from build123d import *

# Parameters (mm, degrees)
SKETCH_1_W                     = 31
SKETCH_1_H                     = 40
SKETCH_1_R                     = 1.6
EXTRUDE_1_DEPTH                = 5
SKETCH_2_W                     = 31
SKETCH_2_H                     = 9.8
EXTRUDE_3_DEPTH                = 8
SKETCH_13_R                    = 1
CUT_EXTRUDE_7_DEPTH            = 5
EXTRUDE_START                  = 1
SKETCH_14_R                    = 3
SKETCH_14_R_2                  = 1
EXTRUDE_8_DEPTH                = 1
HOLE_WIZARD_M3_3_D             = 2.5
HOLE_WIZARD_M3_3_DEPTH         = 6.5
HOLE_WIZARD_M3_3_TIP           = 0.751075774
SKETCH_18_W                    = 31
SKETCH_18_H                    = 3
EXTRUDE_9_DEPTH                = 10
SKETCH_29_W                    = 31
SKETCH_29_H                    = 6.8
EXTRUDE_11_DEPTH               = 2
SKETCH_20_R                    = 1
CUT_EXTRUDE_9_DEPTH            = 9
HOLE_START                     = -9
HOLE_WIZARD_M3_1_OUTLINE_R     = 1.25
HOLE_WIZARD_M3_1_OUTLINE_R_2   = 1
HOLE_WIZARD_M3_1_DEPTH         = 9
HOLE_WIZARD_M3_1_3_D           = 3.2
HOLE_WIZARD_M3_1_3_CBORE_D     = 6
HOLE_WIZARD_M3_1_3_CBORE_DEPTH = 3.1
HOLE_START_2                   = -40
HOLE_WIZARD_M3_2_OUTLINE_R     = 1.25
HOLE_WIZARD_M3_2_OUTLINE_R_2   = 1
HOLE_WIZARD_M3_2_DEPTH         = 9
SKETCH_30_W                    = 31
SKETCH_30_H                    = 7
CUT_EXTRUDE_10_DEPTH           = 4
FILLET_3_R                     = 1


# Read off the part's stored shape, not the designer's step: M3 螺纹孔1, M3 螺纹孔2
with BuildPart() as part:
    # 草图1 → 凸台-拉伸1 (new body)
    with BuildSketch(Plane(origin=(0, 0, 0), x_dir=(1, 0, 0), z_dir=(0, 1, 0))):
        with Locations((15.5, 20)):
            Rectangle(SKETCH_1_W, SKETCH_1_H)
        with Locations(Location((20.5, 27.5, 0), (0, 0, 270))):
            Circle(SKETCH_1_R, mode=Mode.SUBTRACT)
        with Locations(Location((10.5, 27.5, 0), (0, 0, 270))):
            Circle(SKETCH_1_R, mode=Mode.SUBTRACT)
        with Locations(Location((10.5, 12.5, 0), (0, 0, 90))):
            Circle(SKETCH_1_R, mode=Mode.SUBTRACT)
        with Locations(Location((20.5, 12.5, 0), (0, 0, 90))):
            Circle(SKETCH_1_R, mode=Mode.SUBTRACT)
    extrude(amount=EXTRUDE_1_DEPTH)

    # 草图2 → 凸台-拉伸3 (add)
    with BuildSketch(Plane(origin=(0, 0, 0), x_dir=(1, 0, 0), z_dir=(0, 1, 0))):
        with Locations((15.5, 35.1)):
            Rectangle(SKETCH_2_W, SKETCH_2_H)
    extrude(amount=-EXTRUDE_3_DEPTH)

    # 草图13 → 切除-拉伸7 (cut)
    with BuildSketch(Plane.XZ.offset(8)):
        with Locations(Location((15.5, -35.1, 0), (0, 0, 270))):
            Circle(SKETCH_13_R)
    extrude(amount=-CUT_EXTRUDE_7_DEPTH, mode=Mode.SUBTRACT)

    # 草图14 → 凸台-拉伸8 (add)
    with BuildSketch(Plane.XZ.offset(8).offset(EXTRUDE_START)):
        with Locations(Location((15.5, -35.1, 0), (0, 0, 270))):
            Circle(SKETCH_14_R)
        with Locations(Location((15.5, -35.1, 0), (0, 0, 270))):
            Circle(SKETCH_14_R_2, mode=Mode.SUBTRACT)
    extrude(amount=-EXTRUDE_8_DEPTH)

    # M3 螺纹孔3
    with Locations(Plane(origin=(0, -9, 0), x_dir=(-1, 0, 0), z_dir=(0, -1, 0))):
        with Locations((-15.5, 35.1)):
            Hole(HOLE_WIZARD_M3_3_D / 2, depth=HOLE_WIZARD_M3_3_DEPTH)
            with Locations((0, 0, -(HOLE_WIZARD_M3_3_DEPTH + HOLE_WIZARD_M3_3_TIP / 2))):  # 118° drill point
                Cone(0, HOLE_WIZARD_M3_3_D / 2, HOLE_WIZARD_M3_3_TIP, mode=Mode.SUBTRACT)

    # 草图18 → 凸台-拉伸9 (add)
    with BuildSketch(Plane(origin=(0, 5, 0), x_dir=(1, 0, 0), z_dir=(0, 1, 0))):
        with Locations((15.5, 8.3)):
            Rectangle(SKETCH_18_W, SKETCH_18_H)
    extrude(amount=-EXTRUDE_9_DEPTH)

    # 草图29 → 凸台-拉伸11 (add)
    with BuildSketch(Plane.XZ):
        with Locations((15.5, -3.4)):
            Rectangle(SKETCH_29_W, SKETCH_29_H)
    extrude(amount=EXTRUDE_11_DEPTH)

    # 草图20 → 切除-拉伸9 (cut)
    with BuildSketch(Plane.XY):
        with Locations((7.5, 2)):
            Circle(SKETCH_20_R)
        with Locations(Location((23.5, 2, 0), (0, 0, 180))):
            Circle(SKETCH_20_R)
    cut_extrude_9 = extrude(amount=-CUT_EXTRUDE_9_DEPTH, mode=Mode.SUBTRACT)

    # Hole Wizard M3 _1 outline → Hole Wizard M3 _1 (cut)
    with BuildSketch(Plane.XY.offset(HOLE_START)):
        with Locations((23.5, 2)):
            Circle(HOLE_WIZARD_M3_1_OUTLINE_R)
        with Locations((23.5, 2)):
            Circle(HOLE_WIZARD_M3_1_OUTLINE_R_2, mode=Mode.SUBTRACT)
    extrude(amount=HOLE_WIZARD_M3_1_DEPTH, mode=Mode.SUBTRACT)

    # Hole Wizard M3 _1 2 outline → Hole Wizard M3 _1 2 (revolve, cut)
    with BuildSketch(Plane(origin=(7.5, 2, 0), x_dir=(1, 0, 0), z_dir=(0, -1, 0))):
        Polygon((0, -9), (0, -9.751075774), (1.25, -9), (1.25, 0), (1, 0), (1, -9), align=None)
    revolve(axis=Axis((7.5, 2, 0), (0, 0, 1)), mode=Mode.SUBTRACT)

    # 镜向1: 切除-拉伸9 across plane
    add(cut_extrude_9.mirror(Plane.XY.offset(-20)), mode=Mode.SUBTRACT)

    # Hole Wizard M3 _1 3 (through all)
    with Locations(Plane(origin=(0, 5, 0), x_dir=(1, 0, 0), z_dir=(0, 1, 0))):
        with Locations((10.5, 27.5), (10.5, 12.5), (20.5, 12.5), (20.5, 27.5)):
            CounterBoreHole(HOLE_WIZARD_M3_1_3_D / 2, HOLE_WIZARD_M3_1_3_CBORE_D / 2, HOLE_WIZARD_M3_1_3_CBORE_DEPTH)

    # M3 螺纹孔2 outline → M3 螺纹孔2 (cut)
    with BuildSketch(Plane.XY.offset(HOLE_START_2)):
        with Locations((7.5, 2)):
            Circle(HOLE_WIZARD_M3_2_OUTLINE_R)
        with Locations((7.5, 2)):
            Circle(HOLE_WIZARD_M3_2_OUTLINE_R_2, mode=Mode.SUBTRACT)
    extrude(amount=HOLE_WIZARD_M3_2_DEPTH, mode=Mode.SUBTRACT)

    # Hole Wizard M3 _2 2 outline → Hole Wizard M3 _2 2 (revolve, cut)
    with BuildSketch(Plane(origin=(23.5, 2, 0), x_dir=(1, 0, 0), z_dir=(0, -1, 0))):
        Polygon((1.25, -31), (0, -30.248924226), (0, -31), (1, -31), (1, -40), (1.25, -40), align=None)
    revolve(axis=Axis((23.5, 2, 0), (0, 0, 1)), mode=Mode.SUBTRACT)

    # 草图30 → 切除-拉伸10 (cut)
    with BuildSketch(Plane.XY):
        with Locations((15.5, 1.5)):
            Rectangle(SKETCH_30_W, SKETCH_30_H)
    cut_extrude_10 = extrude(amount=-CUT_EXTRUDE_10_DEPTH, mode=Mode.SUBTRACT)

    # 镜向3: 切除-拉伸10 across plane
    add(cut_extrude_10.mirror(Plane.XY.offset(-20)), mode=Mode.SUBTRACT)

    # 圆角3
    fillet_3_edges = [part.edges().sort_by_distance(p)[0] for p in [
        (31, 1.5, -4),
        (0, 1.5, -4),
        (31, -5, -40),
        (0, -5, -40),
        (0, 1.5, -36),
        (31, 1.5, -36),
        (31, -5, -8.3),
        (0, -5, -8.3),
    ]]
    fillet(fillet_3_edges, radius=FILLET_3_R)


solid = part.part
The listing builds one solid part. Answer for the finished solid, in the listing's coordinates (mm). A direction names the side the tool comes from. Give positions to 0.01 mm unless a question says otherwise; leave off trailing zeros. Write each loop counter-clockwise with the first axis right and the second up, starting at its lowest first coordinate (ties: lowest second). Pieces come first, ordered by that corner, then holes.
Item 1: Section C-C, the plane y = -6 is taken. Write down the section's boundary in (x, z).
Item 2: Find the intervals of material crossed by line 1 along X through (y, z) = (3.45, -12.5); line 2 along X through (y, z) = (1.05, -27.5); line 3 along Z through (x, y) = (10.5, 2.8), in increasing order.
Item 3: Determine the mould class of faces 5 (the cylindrical face through (6.25, 2.05, -6.46)), 6 (the cylindrical face through (30.699, -5.042, -39.715)), 7 (the cylindrical face through (21.58, 0.94, -28.68)) for opening direction Z: released by +Z, released by -Z, zero draft, split by the parting line, or undercut.
Item 4: Flat-ended cylindrical pins translate along their axes: P1, Ø1, axis at x = 7.5, y = -1, coming from the -Z side; P2, Ø10, axis at x = 16, z = -23.5, coming from the -Y side; P3, Ø0.8, axis at x = 17.5, z = -5.5, coming from the -Y side. Find the tip coordinate at first contact, or state that the pin passes through.
Item 5: Section B-B, the plane z = -12.5 is taken. Write down the section's boundary in (x, y), plus the area to 3 significant figures.
Item 6: Which of the six approach directions +Z, -Z, +X, -X, +Y, -Y give full straight-line access (tool end or side, diameter ignored) to faces 1 (the flat face through (15, -2, -9.8)), 2 (the cylindrical face through (30.699, -4.715, -8.321)), 3 (the flat face through (15, -2, -5)), 4 (the cylindrical face through (6.25, 2.05, -33.53))?
Item 7: Section A-A, the plane x = 20.5 is taken. Write down the section's boundary in (y, z), plus the area to 3 significant figures.
Item 8: Section D-D, the plane x = 27.5 is taken. Write down the section's boundary in (y, z), plus the area to 3 significant figures.
Completed:
1. outline: (0, -39) arc R1 ccw to (1, -40) - (30, -40) arc R1 ccw to (31, -39) - (31, -30.2) - (0, -30.2) - close; hole circle Ø2.5 at (15.5, -35.1)
2. line 1: x = 0 to 7.5, 13.5 to 17.5, 23.5 to 31
2. line 2: x = 0 to 8.9, 12.1 to 18.9, 22.1 to 31
2. line 3: z = -36 to -30.5, -24.5 to -15.5, -9.5 to -4
3. face 5: zero draft
3. face 6: released by -Z
3. face 7: undercut
4. P1: stops at z = -36
4. P2: stops at y = 0
4. P3: stops at y = -2
5. outline: (0, 0) - (8.9, 0) - (8.9, 1.9) - (7.5, 1.9) - (7.5, 5) - (0, 5) - close; (12.1, 0) - (18.9, 0) - (18.9, 1.9) - (17.5, 1.9) - (17.5, 5) - (13.5, 5) - (13.5, 1.9) - (12.1, 1.9) - close; (22.1, 0) - (31, 0) - (31, 5) - (23.5, 5) - (23.5, 1.9) - (22.1, 1.9) - close
5. area: 106 mm2
6. face 1: +X, -X, -Y
6. face 2: +Z, +X, -Y
6. face 3: +Z, +X, -X, -Y
6. face 4: -Z
7. outline: (-8, -40) - (-2, -40) - (-2, -36) - (5, -36) - (5, -30.5) - (1.9, -30.5) - (1.9, -29.1) - (0, -29.1) - (0, -30.2) - (-8, -30.2) - close; (-5, -9.8) - (0, -9.8) - (0, -10.9) - (1.9, -10.9) - (1.9, -9.5) - (5, -9.5) - (5, -4) - (-2, -4) - (-2, -6.8) - (-5, -6.8) - close; (0, -25.9) - (1.9, -25.9) - (1.9, -24.5) - (5, -24.5) - (5, -15.5) - (1.9, -15.5) - (1.9, -14.1) - (0, -14.1) - close
7. area: 202 mm2
8. outline: (-8, -40) - (-2, -40) - (-2, -36) - (5, -36) - (5, -4) - (-2, -4) - (-2, -6.8) - (-5, -6.8) - (-5, -9.8) - (0, -9.8) - (0, -30.2) - (-8, -30.2) - close
8. area: 251 mm2
